Source: CAD feature listing. Evaluate the final solid. Frame: model axes, mm. A direction names the side the tool comes from. Give positions to 0.01 mm unless a question says otherwise; leave off trailing zeros. Write each loop counter-clockwise with the first axis right and the second up, starting at its lowest first coordinate (ties: lowest second). Pieces come first, ordered by that corner, then holes. Notation, with made-up numbers: (83.25, 67) - (93.25, 67) arc R21 ccw to (93.25, 88) - close; hole circle Ø6 at (13, -21.5). An arc over 180 degrees is marked (long way). One line per question, with ' | ' between items. Start each with the question number.
(1) Draft query along X for faces 5 (the cylindrical face through (101.143, -74.289, -114.804)), 6 (the flat face through (51, -75, -50)), 7 (the cylindrical face through (153.573, -65.164, -128.86)). Return one class per face: +X half, -X half, draft (parallel to the pull), parting line (faces both ways), or undercut.
(2) Section B-B, the plane z = -47.5. Return loops of the section in (x, y), plus the area to 3 significant figures.
(3) Section D-D, the plane y = -30. State how many separate pieces and enclosed holes the cut face has, plus the area to 3 significant figures.
(4) Access query for faces 1 (the flat face through (-32, -44, -114)), 2 (the flat face through (25, -75, -50)), 3 (the cylindrical face through (-25.857, -1.711, -114.804)), 4 (the flat face through (0, -64, -69)). Directions: +Z, -Z, +X, -X, +Y, -Y. A direction counts if a zero-diameter tool reaches every point of the face in a straight line with its end or side. Return the directions, or none.
(5) Section C-C, the plane x = -13. Return loops of the section in (y, z).
(6) Pin query (flat end, axial travel): pin 1 (1 mm diameter, centred on y = -113, z = -100.5, fed in from +X); pin 2 (6 mm diameter, centred on x = -38, z = -127.5, fed in from -Y). Return the tip coordinate at first contact, or that it passes through.
(7) Section A-A, the plane y = -85.5. Return loops of the section in (x, z), plus the area to 3 significant figures.
(8) Ray query, line 1 (X direction, y = -117.5, z = -80.5); line 2 (Z direction, x = 93.5, y = -36); line 3 (X direction, y = -15.5, z = -67). Return the intervals inside material, ascending. Write a range as [from, to].
```python
from build123d import *

# Parameters (mm, degrees)
F0_W      = 127
F0_H      = 139
F1_DEPTH  = 76
F3_W      = 76
F3_H      = 26
F4_DEPTH  = 51
F2_W      = 76
F2_H      = 26
F5_DEPTH  = 51
F6_DEPTH  = 38
F7_DEPTH  = 38
F8_R      = 19
F9_DEPTH  = 26.001
F10_R     = 37.99999
F11_R     = 28.5
F11_R_2   = 19
F13_DEPTH = 1
F12_R     = 28.5
F12_R_2   = 19
F14_DEPTH = 1
F15_R     = 6
F17_DEPTH = 165.001
F18_W     = 26
F18_H     = 125.8650070512
F21_DEPTH = 18.3847763109
F22_DEPTH = 26.8710576851
F23_DEPTH = 35.3563390593


# Not quite as in the source:
# - a fillet or chamfer is up to 0.001 mm smaller than in the source, because OpenCascade refuses the exact size


with BuildPart() as f1:
    # F0 (on Right) → F1 (new body)
    with BuildSketch(Plane.YZ):
        with Locations((-63.5, -69.5)):
            Rectangle(F0_W, F0_H)
    extrude(amount=F1_DEPTH)

    # F3 (on face) → F4 (join)
    with BuildSketch(Plane.YZ.offset(76)):
        with Locations((-38, -126)):
            Rectangle(F3_W, F3_H)
    extrude(amount=F4_DEPTH)

    # F2 (on face) → F5 (join)
    with BuildSketch(Plane(origin=(0, 0, 0), x_dir=(0, -1, 0), z_dir=(-1, 0, 0))):
        with Locations((38, -126)):
            Rectangle(F2_W, F2_H)
    extrude(amount=F5_DEPTH)

    # F6 (add): a face of the model
    f6_faces = [f1.faces().sort_by_distance(p)[0] for p in [
        (-51, -38, -126),
    ]]
    extrude(f6_faces, amount=F6_DEPTH)

    # F7 (add): a face of the model
    f7_faces = [f1.faces().sort_by_distance(p)[0] for p in [
        (127, -38, -126),
    ]]
    extrude(f7_faces, amount=F7_DEPTH)

    # F8 (on face) → F9 (cut, through all)
    with BuildSketch(Plane.XY.offset(-113)):
        with Locations((-51, -38)):
            Circle(F8_R)
        with Locations((127, -38)):
            Circle(F8_R)
    extrude(amount=-F9_DEPTH, mode=Mode.SUBTRACT)

    # F10 (radius 38 in the source; OpenCascade refuses exactly that, so slightly less here)
    f10_edges = [f1.edges().sort_by_distance(p)[0] for p in [
        (-89, 0, -126),
        (-89, -76, -126),
        (165, -76, -126),
        (165, 0, -126),
    ]]
    fillet(f10_edges, radius=F10_R)

    # F11 (on face) → F13 (cut)
    with BuildSketch(Plane.XY.offset(-113)):
        with Locations((-51, -38)):
            Circle(F11_R)
        with Locations((-51, -38)):
            Circle(F11_R_2, mode=Mode.SUBTRACT)
    extrude(amount=-F13_DEPTH, mode=Mode.SUBTRACT)

    # F12 (on face) → F14 (cut)
    with BuildSketch(Plane.XY.offset(-113)):
        with Locations((127, -38)):
            Circle(F12_R)
        with Locations((127, -38)):
            Circle(F12_R_2, mode=Mode.SUBTRACT)
    extrude(amount=-F14_DEPTH, mode=Mode.SUBTRACT)

    # F15
    f15_edges = [f1.edges().sort_by_distance(p)[0] for p in [
        (-25.500005, -76, -113),
        (-77.870061, -11.129939, -113),
        (101.500005, -76, -113),
    ]]
    fillet(f15_edges, radius=F15_R)

    # F16 (on face) → F17 (cut, through all)
    with BuildSketch(Plane(origin=(0, 0, 0), x_dir=(0, -1, 0), z_dir=(-1, 0, 0))):
        Polygon((127, 0), (38, 0), (127, -89), align=None)
    extrude(amount=-F17_DEPTH, mode=Mode.SUBTRACT)

    # F18 (on face) → F21 (cut, through all)
    with BuildSketch(Plane(origin=(0, -19, 19), x_dir=(1, 0, 0), z_dir=(0, -0.7071067812, 0.7071067812))):
        with Locations((38, -89.8025612107)):
            Rectangle(F18_W, F18_H)
    extrude(amount=-F21_DEPTH, mode=Mode.SUBTRACT)

    # F22 (cut, through all): a face of the model
    f22_faces = [f1.faces().sort_by_distance(p)[0] for p in [
        (38, -31.5, -6.5),
    ]]
    extrude(f22_faces, amount=-F22_DEPTH, mode=Mode.SUBTRACT)

    # F23 (cut, through all): a face of the model
    f23_faces = [f1.faces().sort_by_distance(p)[0] for p in [
        (38, -120.5, -95.5),
    ]]
    extrude(f23_faces, amount=-F23_DEPTH, mode=Mode.SUBTRACT)


solid = f1.part
```
Check sheet entries:
1) face 5: draft | face 6: undercut | face 7: +X half
2) outline: (0, -85.5) - (25, -85.5) - (25, -59.5) - (51, -59.5) - (51, -85.5) - (76, -85.5) - (76, 0) - (0, 0) - close | area: 5,820 mm²
3) separate pieces: 3 | enclosed holes: 0 | area: 12,800 mm²
4) face 1: +Z | face 2: +Z, -Y | face 3: +Z, -X, +Y | face 4: +Z, -X, -Y
5) outline: (-76, -139) - (0, -139) - (0, -119) arc R6 ccw to (-6, -113) - (-70, -113) arc R6 ccw to (-76, -119) - close
6) pin 1: x = 76 | pin 2: y = -76
7) outline: (0, -139) - (76, -139) - (76, -47.5) - (51, -47.5) - (51, -73.5) - (25, -73.5) - (25, -47.5) - (0, -47.5) - close | area: 6,280 mm²
8) line 1: [0, 25], [51, 76] | line 2: [-139, -113] | line 3: [0, 76]
